Part print with two shaded views. Sizes in mm from the minimum x, y, z corner. Give positions to 0.01 mm unless a question says otherwise; leave off trailing zeros. Order: outer loops, then holes, each group sorted by start corner. A loop starts at its lowest first (then second) coordinate and runs counter-clockwise, first axis right, second up. Notation, with made-up numbers: M -13.5,50.25 L 9.5,50.25 A14 cw 9.5,60.25 Z; hole C 53.5,16 d8. An arc over 180 degrees is marked long. Return JSON: item names as keys, results as strings. Group by question number.
1. Wall check: probe 1 along X at (y, z) = (1.65, 38.5); probe 2 along Z at (x, y) = (25.4, 1.7); probe 3 along Z at (x, y) = (29, 2.35). Give the ranges that are in metal, low to high. Write a range as [from, to].
2. Slice it at A-A on z = 38.1. List the corners of the cut face in (x, y), then the cut area to 3 significant figures.
3. Slice it at B-B on x = 25.4. List the corners of the cut face in (y, z).
4. Pin check, flat tips, straight feed: pin 1 (8 mm diameter, centred on x = 95.5, z = 52.5, fed in from -Y); pin 2 (3 mm diameter, centred on x = 129.5, z = 37, fed in from -Y). Stop position of each tip, or through.
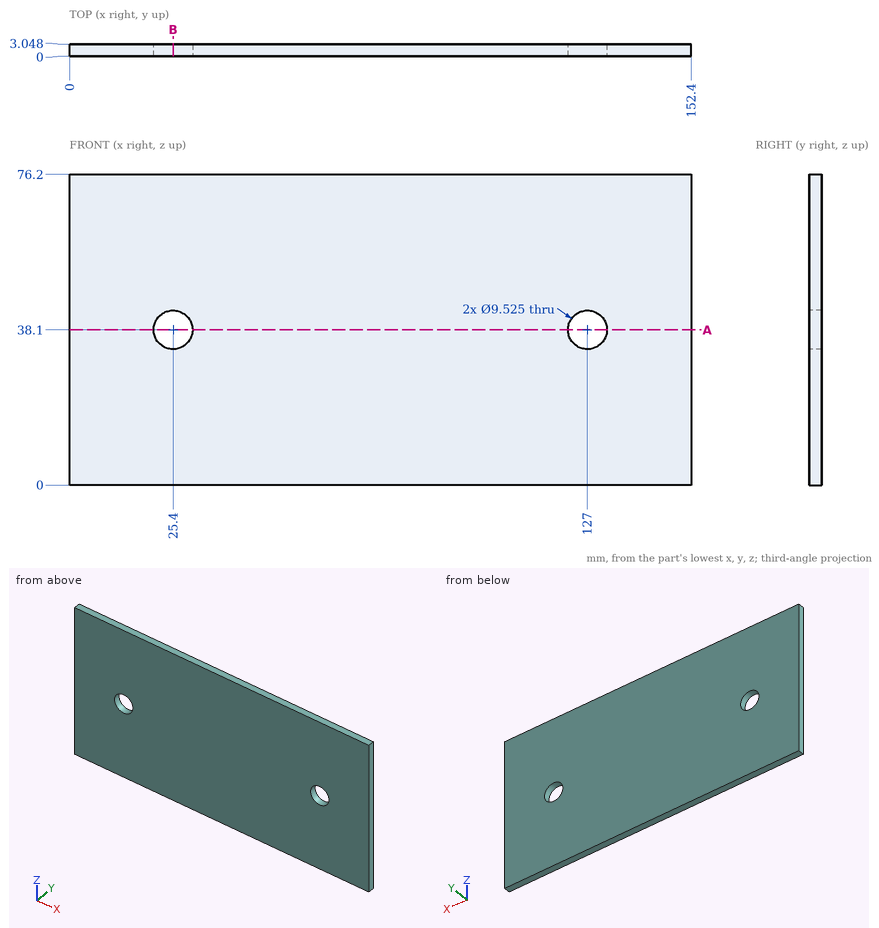
Result:
{
 "1": {"probe 1": "x = [0, 20.65], [30.15, 122.25], [131.75, 152.4]", "probe 2": "z = [0, 33.34], [42.86, 76.2]", "probe 3": "z = [0, 34.98], [41.22, 76.2]"},
 "2": {"outline": "M 0,0 L 20.64,0 L 20.64,3.05 L 0,3.05 Z; M 30.16,0 L 122.24,0 L 122.24,3.05 L 30.16,3.05 Z; M 131.76,0 L 152.4,0 L 152.4,3.05 L 131.76,3.05 Z", "area": "406 mm2"},
 "3": {"outline": "M 0,0 L 3.05,0 L 3.05,33.34 L 0,33.34 Z; M 0,42.86 L 3.05,42.86 L 3.05,76.2 L 0,76.2 Z"},
 "4": {"pin 1": "stops at y = 0", "pin 2": "passes through"}
}
